Could you check a few things on this drawing? It's one solid part, dimensions in mm from its lowest x, y, z. A direction names the side the tool comes from. Give positions to 0.01 mm unless a question says otherwise; leave off trailing zeros. Loops run counter-clockwise (first coordinate to the right, second up) from the corner with the lowest first, then second, coordinate; pieces in that order, holes last.
1. Imagine slicing it at A-A (y = 25.4). Count the separate pieces of the cut face and the enclosed holes in it.
2. For P1, Ø10, axis at y = 14.5, z = 21, coming from the +X side; P2, Ø8, axis at x = 61.5, y = 44, coming from the +Z side, each with a flat end and sliding along its axis, tell me the tip position at first contact or that it passes through.
3. Imagine slicing it at B-B (y = 15). List the corners of the cut face in (x, z) for me.
4. For the marked faces 1 and 2, which set-ups out of +Z, -Z, +X, -X, +Y, -Y let a thin tool reach every point of the face, with its end or its side?
5. Imagine slicing it at D-D (z = 19). List the corners of the cut face in (x, y) for me.
6. I need wall thicknesses on line 1 along X through (y, z) = (7, 65); line 2 along Z through (x, y) = (14, 14.5); line 3 along Z through (x, y) = (8, 6). Which ranges of each line are inside material? Lowest first, please.
7. Imagine slicing it at C-C (x = 35). List the corners of the cut face in (y, z) for me.
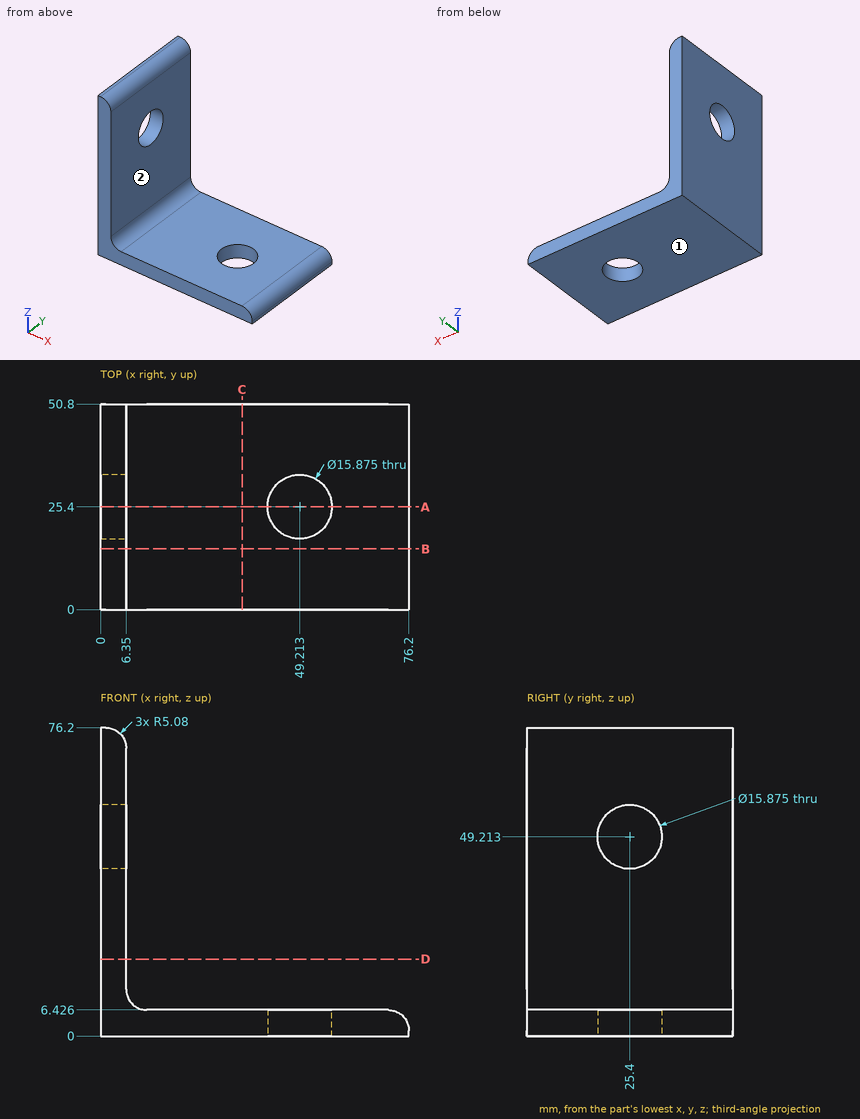
Derived:
1. separate pieces: 3
1. enclosed holes: 0
2. P1: stops at x = 6.35
2. P2: stops at z = 6.43
3. outline: (0, 0) - (76.2, 0) - (76.2, 1.35) arc R5.08 ccw to (71.12, 6.43) - (11.43, 6.43) arc R5.08 cw to (6.35, 11.51) - (6.35, 71.12) arc R5.08 ccw to (1.27, 76.2) - (0, 76.2) - close
4. face 1: -Z, +X, -X, +Y, -Y
4. face 2: +Z, +X, +Y, -Y
5. outline: (0, 0) - (6.35, 0) - (6.35, 50.8) - (0, 50.8) - close
6. line 1: x = 0 to 6.35
6. line 2: z = 0 to 6.43
6. line 3: z = 0 to 7.76
7. outline: (0, 0) - (50.8, 0) - (50.8, 6.43) - (0, 6.43) - close
